from build123d import *

# Parameters (mm, degrees)
BASES_W            = 20
BASES_H            = 40
BASE_DEPTH         = 10.25
BASE_F_R           = 1
CUT_EXTRUDE3_DEPTH = 31.335622624


with BuildPart() as part:
    # BaseS → BASE (new, symmetric)
    with BuildSketch(Plane(origin=(0, 0, 0), x_dir=(1, 0, 0), z_dir=(0, 1, 0))):
        Rectangle(BASES_W, BASES_H)
    extrude(amount=BASE_DEPTH, both=True)

    # BASE F
    base_f_edges = [part.edges().sort_by_distance(p)[0] for p in [
        (10, 0, 20),
        (-10, 0, 20),
        (-10, 0, -20),
        (10, 0, -20),
    ]]
    fillet(base_f_edges, radius=BASE_F_R)

    # PocketS → Cut-Extrude3 (cut, through all)
    with BuildSketch(Plane(origin=(0, 10.25, 0), x_dir=(1, 0, 0), z_dir=(0, 1, 0))):
        with BuildLine():
            Line((9, 19.2), (-9, 19.2))
            ThreePointArc((-9, 19.2), (-9.141421356, 19.141421356), (-9.2, 19))
            Line((-9.2, 19), (-9.2, -19))
            ThreePointArc((-9.2, -19), (-9.141421356, -19.141421356), (-9, -19.2))
            Line((-9, -19.2), (9, -19.2))
            ThreePointArc((9, -19.2), (9.141421356, -19.141421356), (9.2, -19))
            Line((9.2, -19), (9.2, 19))
            ThreePointArc((9.2, 19), (9.141421356, 19.141421356), (9, 19.2))
        make_face()
    extrude(amount=-CUT_EXTRUDE3_DEPTH, mode=Mode.SUBTRACT)


solid = part.part
Work out the finished part from the listing and answer in its coordinate system (mm). A direction names the side the tool comes from. Give positions to 0.01 mm unless a question says otherwise; leave off trailing zeros. Write each loop counter-clockwise with the first axis right and the second up, starting at its lowest first coordinate (ties: lowest second). Pieces come first, ordered by that corner, then holes.
Q1. The part is cut by section B-B on x = -5. Give the vertices of the cut face in (y, z).
Answer:
outline: (-10.25, -20) - (10.25, -20) - (10.25, -19.2) - (-10.25, -19.2) - close; (-10.25, 19.2) - (10.25, 19.2) - (10.25, 20) - (-10.25, 20) - close
Q2. The part is cut by section A-A on z = -4.5. Give the vertices of the cut face in (x, y).
Answer:
outline: (-10, -10.25) - (-9.2, -10.25) - (-9.2, 10.25) - (-10, 10.25) - close; (9.2, -10.25) - (10, -10.25) - (10, 10.25) - (9.2, 10.25) - close
Q3. The part is cut by section C-C on y = 3.5. Give the vertices of the cut face in (x, z), and give its area (3 significant figures).
Answer:
outline: (-10, -19) arc R1 ccw to (-9, -20) - (9, -20) arc R1 ccw to (10, -19) - (10, 19) arc R1 ccw to (9, 20) - (-9, 20) arc R1 ccw to (-10, 19) - close; hole (-9.2, -19) arc R0.2 ccw to (-9, -19.2) - (9, -19.2) arc R0.2 ccw to (9.2, -19) - (9.2, 19) arc R0.2 ccw to (9, 19.2) - (-9, 19.2) arc R0.2 ccw to (-9.2, 19) - close
area: 92.6 mm2
Q4. For a pull along X with two mould halves and no side action, classify faces 3 (the face through (-9.715, -0.143, -19.699)), 4 (the face through (9.2, 0, 0)), 5 (the face through (9.715, -0.143, -19.699)) as released by +X, released by -X, zero draft, split by the parting line, or undercut.
Answer:
face 3: released by -X
face 4: undercut
face 5: released by +X
Q5. Straight lines are drawn through the part: L1, parallel to Z at x = -1, y = -2.25; L2, parallel to X at y = -8.25, z = -2.5. For each, find the intervals that lie inside material, in ascending order.
Answer:
L1: z = -20 to -19.2, 19.2 to 20
L2: x = -10 to -9.2, 9.2 to 10
Q6. A tool of negligible diameter and unlimited length cuts with its end or side. For faces 1 (the face through (9.715, 0.143, 19.699)), 2 (the face through (0, 0, -19.2)), from which of +Z, -Z, +X, -X, +Y, -Y can it reach the whole face along a straight path? Write none if from no direction.
Answer:
face 1: +Z, +X, +Y, -Y
face 2: +Y, -Y
